```python
from build123d import *
from OCP.BRepFilletAPI import BRepFilletAPI_MakeFillet

# Parameters (mm, degrees)
SCHIZZO2_R                   = 1.575
SCHIZZO2_R_2                 = 1.525
ESTRUSIONE_ESTRUSIONE1_DEPTH = 1.5
RACCORDO1_R1                 = 3
RACCORDO1_R2                 = 10
ESTRUSIONE_ESTRUSIONE2_START = -1.5
SCHIZZO4_R                   = 1.55
ESTRUSIONE_ESTRUSIONE2_DEPTH = 2.5
ESTRUSIONE_ESTRUSIONE3_START = 2.5
ESTRUSIONE_ESTRUSIONE3_DEPTH = 2.5


with BuildPart() as part:
    # Schizzo2 → Estrusione-Estrusione1 (new body)
    with BuildSketch(Plane.XY):
        Polygon((10.835450111, 45.456844872), (10.835450111, 104.878132603), (-7.726239407, 141.30749945), (4.747851932, 147.663366447), (24.835450111, 108.23923523), (24.835450111, 45.456844872), align=None)
        with Locations((17.835450111, 52.456844872)):
            Circle(SCHIZZO2_R, mode=Mode.SUBTRACT)
        with Locations((1.688739761, 138.248387279)):
            Circle(SCHIZZO2_R_2, mode=Mode.SUBTRACT)
        with Locations((7.590616257, 126.665302465)):
            Circle(SCHIZZO2_R_2, mode=Mode.SUBTRACT)
    extrude(amount=ESTRUSIONE_ESTRUSIONE1_DEPTH)

    # Raccordo1: one fillet with a radius per group of edges: ONE call of the kernel's fillet builder (fillet() takes one radius for all edges)
    raccordo1_edges_1 = [part.edges().sort_by_distance(p)[0] for p in [
        (4.747851932, 147.663366447, 0.75),
        (-7.726239407, 141.30749945, 0.75),
        (10.835450111, 45.456844872, 0.75),
        (24.835450111, 45.456844872, 0.75),
    ]]
    raccordo1_edges_2 = [part.edges().sort_by_distance(p)[0] for p in [
        (24.835450111, 108.23923523, 0.75),
        (10.835450111, 104.878132603, 0.75),
    ]]
    raccordo1 = BRepFilletAPI_MakeFillet(part.part.solid().wrapped)
    for e in raccordo1_edges_1:
        raccordo1.Add(RACCORDO1_R1, e.wrapped)
    for e in raccordo1_edges_2:
        raccordo1.Add(RACCORDO1_R2, e.wrapped)
    add(Compound.cast(raccordo1.Shape()), mode=Mode.REPLACE)

    # Schizzo4 → Estrusione-Estrusione2 (add)
    with BuildSketch(Plane(origin=(0, 0, 0), x_dir=(-1, 0, 0), z_dir=(0, 0, -1)).offset(ESTRUSIONE_ESTRUSIONE2_START)):
        with Locations(Location((-13.532140626, 53.421016786, 0), (0, 0, 180))):
            Circle(SCHIZZO4_R)
        with Locations(Location((-22.138759596, 51.492672958, 0), (0, 0, 180))):
            Circle(SCHIZZO4_R)
    extrude(amount=-ESTRUSIONE_ESTRUSIONE2_DEPTH)

    # Schizzo5 → Estrusione-Estrusione3 (add)
    with BuildSketch(Plane.XY.offset(1.5).offset(ESTRUSIONE_ESTRUSIONE3_START)):
        with BuildLine():
            Line((24.835450111, 59.217112451), (14.402001203, 59.217112451))
            add(Edge.make_bspline(
                [(14.402001203, 59.217112451), (13.28177849, 59.164141407), (11.913165696, 58.833942628), (10.835450111, 58.162340852)],
                knots=[0, 0, 0, 0, 0.33692331, 0.33692331, 0.33692331, 0.33692331], degree=3))
            Line((10.835450111, 58.162340852), (10.835450111, 102.477345012))
            ThreePointArc((10.835450111, 102.477345012), (10.559149315, 104.811798651), (9.745515353, 107.01725001))
            Line((9.745515353, 107.01725001), (6.567581855, 113.254295679))
            Line((6.567581855, 113.254295679), (8.349594903, 114.162276678))
            Line((8.349594903, 114.162276678), (11.527528401, 107.925231009))
            ThreePointArc((11.527528401, 107.925231009), (12.503889156, 105.278689378), (12.835450111, 102.477345012))
            Line((12.835450111, 102.477345012), (12.835450111, 69.217112451))
            Line((12.835450111, 69.217112451), (22.835450111, 69.217112451))
            Line((22.835450111, 69.217112451), (22.835450111, 105.838447639))
            ThreePointArc((22.835450111, 105.838447639), (22.614409474, 107.70601055), (21.963502304, 109.470371637))
            Line((21.963502304, 109.470371637), (17.259660145, 118.702181676))
            Line((17.259660145, 118.702181676), (19.041673193, 119.610162675))
            Line((19.041673193, 119.610162675), (23.745515353, 110.378352637))
            ThreePointArc((23.745515353, 110.378352637), (24.559149315, 108.172901278), (24.835450111, 105.838447639))
            Line((24.835450111, 105.838447639), (24.835450111, 59.217112451))
        make_face()
    extrude(amount=-ESTRUSIONE_ESTRUSIONE3_DEPTH)


solid = part.part
```
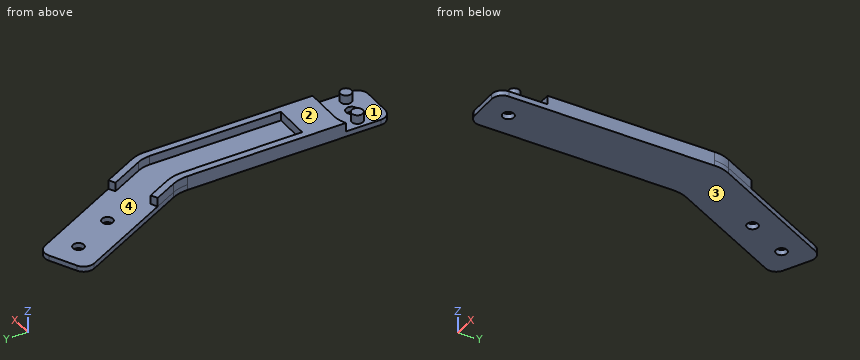
Geometry check sheet. Reference: the model listing, model coordinates, mm. Face numbers are marked on the shaded views. A direction names the side the tool comes from. Give positions to 0.01 mm unless a question says otherwise; leave off trailing zeros. Write each loop counter-clockwise with the first axis right and the second up, starting at its lowest first coordinate (ties: lowest second). Pieces come first, ordered by that corner, then holes. Notation, with made-up numbers: (5.25, 25.5) -> (31.25, 25.5) arc R27 ccw to (31.25, 55.5) -> close; hole circle Ø4 at (-24.75, -0.5). An arc over 180 degrees is marked (long way). Use one line per item in the form item = value.
Item 1: Depth check by flat-ended pin: pin 1 Ø1.2 at (y, z) = (79.5, 2.5) entering from -X; pin 2 Ø12 at (x, y) = (3, 94.5) entering from +Z; pin 3 Ø3 at (x, y) = (19.5, 76.5) entering from -Z; pin 4 Ø3.5 at (x, y) = (1.69, 138.25) entering from +Z. Enter the tip coordinate at first touch or a pass-through.
Results list:
pin_1 = 10.84
pin_2 = through
pin_3 = 0
pin_4 = 1.5
Item 2: Sectioned sample at B-B on x = 4.5. Enter the section's corners in (y, z), plus the area to 3 significant figures.
Results list:
outline = (117.31, 0) -> (146.43, 0) -> (146.43, 1.5) -> (117.31, 1.5) -> close
area = 43.7 mm2
Item 3: Sectioned sample at A-A on z = 2.6. Count the separate pieces of the cut face and the enclosed holes in it, plus the area to 3 significant figures.
Results list:
separate_pieces = 3
enclosed_holes = 0
area = 350 mm2
Item 4: Access from +Z, -Z, +X, -X, +Y, -Y to the whole of each face (thin tool, end or side, straight path). Record for the marked faces 1 and 2.
Results list:
face_1 = +Z
face_2 = +Z, +X, -X, +Y, -Y
Item 5: Mould release check, pull along X, two halves, no side actions. Record for the marked faces 3 and 4: released by +X, released by -X, zero draft, split by the parting line, or undercut.
Results list:
face_3 = zero draft
face_4 = undercut
Item 6: Scan lines: line 1 (X direction, y = 86, z = 2.5); line 2 (Y direction, x = 22, z = 3); line 3 (Z direction, x = -2.5, y = 140.5). Record each from-to range of solid material in increasing order.
Results list:
line_1 = 10.84 to 12.84, 22.84 to 24.84
line_2 = 49.95 to 53.04, 59.22 to 69.22, 109.4 to 113.8
line_3 = 0 to 1.5
